from build123d import *

# Parameters (mm, degrees)
F0_W        = 75.0152692199
F0_H        = 43.3505326509
F1_DEPTH    = 127
F2_T        = -2.54
F3_T1_DEPTH = 100.4152692199
F3_T3_DEPTH = 68.7505326509


# Not quite as in the source:
# - a fillet or chamfer that OpenCascade refuses, or shapes differently, is made with other operations: its cross-section is extruded or revolved along the edge and cut away or added


with BuildPart() as f1:
    # F0 (on Top) → F1 (new body)
    with BuildSketch(Plane.XY):
        with Locations((1.8848069012, 0.6596818566)):
            Rectangle(F0_W, F0_H)
    extrude(amount=F1_DEPTH)

    # F2
    f2_openings = [f1.faces().sort_by_distance(p)[0] for p in [
        (1.884807, 0.659682, 127),
    ]]
    offset(amount=F2_T, openings=f2_openings)

    # F3: fillet of radius 5.08 on 4 edges, made by hand

    # F3_s2 → F3_t1 (cut)
    with BuildSketch(Plane.YZ.offset(-48.3228277087)):
        with BuildLine():
            ThreePointArc((22.3349481821, 121.92), (20.8470506305, 125.5121024484), (17.2549481821, 127))
            Line((17.2549481821, 127), (22.3349481821, 127))
            Line((22.3349481821, 127), (22.3349481821, 121.92))
        make_face()
        with BuildLine():
            ThreePointArc((-21.0155844688, 121.92), (-19.5276869173, 125.5121024484), (-15.9355844688, 127))
            Line((-15.9355844688, 127), (-21.0155844688, 127))
            Line((-21.0155844688, 127), (-21.0155844688, 121.92))
        make_face()
    extrude(amount=F3_T1_DEPTH, mode=Mode.SUBTRACT)

    # F3_s4 → F3_t3 (cut)
    with BuildSketch(Plane.XZ.offset(-35.0349481821)):
        with BuildLine():
            ThreePointArc((-35.6228277087, 121.92), (-34.1349301571, 125.5121024484), (-30.5428277087, 127))
            Line((-30.5428277087, 127), (-35.6228277087, 127))
            Line((-35.6228277087, 127), (-35.6228277087, 121.92))
        make_face()
        with BuildLine():
            ThreePointArc((39.3924415112, 121.92), (37.9045439596, 125.5121024484), (34.3124415112, 127))
            Line((34.3124415112, 127), (39.3924415112, 127))
            Line((39.3924415112, 127), (39.3924415112, 121.92))
        make_face()
    extrude(amount=F3_T3_DEPTH, mode=Mode.SUBTRACT)


solid = f1.part
Input: part model. Units: mm. Frame: model coordinates. A direction names the side the tool comes from. Coordinates: 2 decimals unless noted, no trailing zeros. Loops run counter-clockwise (first coordinate to the right, second up) from the corner with the lowest first, then second, coordinate; pieces in that order, holes last. Notation, with made-up numbers: (-27.5, 77) - (-0.5, 77) arc R8 ccw to (-0.5, 83) - close; hole circle Ø5 at (52.25, 25.5). An arc over 180 degrees is marked (long way). Answer in a Markdown table with one row per item. Add a question column.
Item 1: Mould query, pull axis X, two halves, no side actions, for faces 1 (the cylindrical face through (1.36, -20.35, 124.43)), 2 (the flat face through (36.852, 0, 64)), 3 (the cylindrical face through (38.73, 0.96, 124.43)). Classes: released by +X, released by -X, zero draft, split by the parting line, or undercut.
Item 2: Section query C-C on x = -17. Return the cut outline in (y, z).
Item 3: Contact query for a flat-ended pin moving along its axis: P1, Ø4, axis at x = 30.5, y = 12, coming from the +Z side. Output: stop coordinate, or through.
Item 4: Access query for faces 4 (the flat face through (1, 1, 0)), 5 (the flat face through (1, 19.795, 64)). Directions: +Z, -Z, +X, -X, +Y, -Y. A direction counts if a zero-diameter tool reaches every point of the face in a straight line with its end or side. Return the directions, or none.
Item 5: Section query B-B on y = -0.5. Return the cut outline in (x, z), then the cut area to 3 significant figures.
Item 6: Line query: line 1 along X through (y, z) = (8, 69.5); line 2 along Y through (x, z) = (27, 44); line 3 along Z through (x, y) = (0.5, 11.5). Output: solid intervals per line, ascending. Write a range as [from, to].
Item 7: Section query A-A on z = 99.5. Return the cut outline in (x, y).
Recorded:
| question | item | result |
|---|---|---|
| 1 | face 1 | zero draft |
| 1 | face 2 | undercut |
| 1 | face 3 | released by +X |
| 2 | outline | (-21.02, 0) - (22.33, 0) - (22.33, 121.92) arc R5.08 ccw to (19.79, 126.32) - (19.79, 2.54) - (-18.48, 2.54) - (-18.48, 126.32) arc R5.08 ccw to (-21.02, 121.92) - close |
| 3 | P1 | z = 2.54 |
| 4 | face 4 | -Z, +X, -X, +Y, -Y |
| 4 | face 5 | +Z |
| 5 | outline | (-35.62, 0) - (39.39, 0) - (39.39, 121.92) arc R5.08 ccw to (36.85, 126.32) - (36.85, 2.54) - (-33.08, 2.54) - (-33.08, 126.32) arc R5.08 ccw to (-35.62, 121.92) - close |
| 5 | area | 813 mm^2 |
| 6 | line 1 | [-35.62, -33.08], [36.85, 39.39] |
| 6 | line 2 | [-21.02, -18.48], [19.79, 22.33] |
| 6 | line 3 | [0, 2.54] |
| 7 | outline | (-35.62, -21.02) - (39.39, -21.02) - (39.39, 22.33) - (-35.62, 22.33) - close; hole (-33.08, -18.48) - (36.85, -18.48) - (36.85, 19.79) - (-33.08, 19.79) - close |
